```python
from build123d import *

# Parameters (mm, degrees)
SKETCH2_W          = 5.08
SKETCH2_H          = 25.4
CUT_EXTRUDE1_DEPTH = 25.4


with BuildPart() as part:
    # Sketch1 → Revolve1 (revolve)
    with BuildSketch(Plane.XY, mode=Mode.PRIVATE) as revolve1_sk:
        Polygon((0, 14.5034), (25.4, 14.5034), (25.4, 19.05), (0, 26.9875), (0, 25.4), (-25.4, 25.4), (-25.4, 16.0909), (0, 16.0909), align=None)
    revolve(revolve1_sk.sketch.rotate(Axis((-1.27, 0, 0), (1, 0, 0)), 90), axis=Axis((-1.27, 0, 0), (1, 0, 0)))

    # Sketch2 → Cut-Extrude1 (cut)
    with BuildSketch(Plane.ZY.offset(25.4)):
        Polygon((28.76630657, -13.675295474), (6.769261314, -0.975295474), (4.229261314, -5.374704526), (26.22630657, -18.074704526), align=None)
        with Locations((0, 19.05)):
            Rectangle(SKETCH2_W, SKETCH2_H)
        Polygon((-26.22630657, -18.074704526), (-4.229261314, -5.374704526), (-6.769261314, -0.975295474), (-28.76630657, -13.675295474), align=None)
    extrude(amount=-CUT_EXTRUDE1_DEPTH, mode=Mode.SUBTRACT)


solid = part.part
```
Can you work these out from the model? Positions are in its coordinate system, mm. A direction names the side the tool comes from. Give positions to 0.01 mm unless a question says otherwise; leave off trailing zeros. Loops run counter-clockwise (first coordinate to the right, second up) from the corner with the lowest first, then second, coordinate; pieces in that order, holes last. Notation, with made-up numbers: M 37,78 L 91,78 A29 cw 91,103 Z; hole C -12,-15 d11. An arc over 180 degrees is marked long. One line per question, with ' | ' between items. Start each with the question number.
Q1. If we mould it in two halves opening along Z, with no side actions, what happens to faces 1 (the flat face through (-12.878, -8.124, 19.15)), 2 (the cylindrical face through (-12.9, -25.4, 0.3)), 3 (the flat face through (-25.4, -18, 0))? For each: +Z half, -Z half, draft (parallel to the pull), parting line (faces both ways), or undercut.
Q2. If we section it at B-B (z = 0): Please give me the cut outline in (x, y), plus the area to 3 significant figures.
Q3. For pin 1 Ø5 at (x, y) = (-17, 12.5) entering from +Z; pin 2 Ø4 at (x, y) = (-12.5, -14) entering from -Z; pin 3 Ø10 at (x, z) = (7.5, 20) entering from -Y, each with a flat end and sliding along its axis, tell me the tip position at first contact or that it passes through.
Q4. If I drill on line 1 (Z direction, x = -14.5, y = 10); line 2 (Y direction, x = 17, z = 0) (3 decimals); line 3 (Y direction, x = 4, z = 11), over which ranges is the centre line in solid material (lowest first)? Write a range as from..to.
Q5. If we section it at C-C (x = 20): Please give me the cut outline in (y, z) (1 decimal), plus the area to 3 significant figures.
Q6. For faces 4 (the flat face through (-25.4, 11, -17)), 5 (the cylindrical face through (-12.522, 8.218, 13.834)), 6 (the cylindrical face through (-12.88, 12.41, -22.16)), 7 (the cylindrical face through (-12.878, 12.991, 21.827)), 8 (the flat face through (-13, 21, -2.54)), which set-ups out of +Z, -Z, +X, -X, +Y, -Y let a thin tool reach every point of the face, with its end or its side?
Q7. If we section it at A-A (y = 0): Please give me the cut outline in (x, z), plus the area to 3 significant figures.
Computed:
1) face 1: undercut | face 2: parting line | face 3: draft
2) outline: M -25.4,-25.4 L 0,-25.4 L 0,-26.99 L 25.4,-19.05 L 25.4,-14.5 L 0,-14.5 L 0,-16.09 L -25.4,-16.09 Z; M 0,14.5 L 25.4,14.5 L 25.4,19.05 L 0,26.99 Z | area: 669 mm²
3) pin 1: stops at z = 23.35 | pin 2: stops at z = -20.62 | pin 3: stops at y = -20.03
4) line 1: z = -23.35..-12.61, 12.61..23.35 | line 2: y = -21.675..-14.503, 14.503..21.675 | line 3: y = -23.27..-9.45, 9.45..23.27
5) outline: C 0,0 d41.5; hole C 0,0 d29 | area: 690 mm²
6) face 4: +Z, -Z, -X, +Y, -Y | face 5: -X | face 6: -Z, -X | face 7: +Z, -X | face 8: -X, +Y
7) outline: M -25.4,-25.4 L 0,-25.4 L 0,-26.99 L 25.4,-19.05 L 25.4,-14.5 L 0,-14.5 L 0,-16.09 L -25.4,-16.09 Z; M -25.4,16.09 L 0,16.09 L 0,14.5 L 25.4,14.5 L 25.4,19.05 L 0,26.99 L 0,25.4 L -25.4,25.4 Z | area: 905 mm²
